Autodesk Inventor part; units mm, degrees
ref_plane "YZ Plane" through (0, 0, 0) normal (1, 0, 0) x (0, 1, 0)
ref_plane "XZ Plane" through (0, 0, 0) normal (0, 1, 0) x (-1, 0, 0)
ref_plane "XY Plane" through (0, 0, 0) normal (0, 0, 1) x (1, 0, 0)
sketch "スケッチ1" plane through (0, 0, 0) normal (0, 0, 1) x (1, 0, 0)
  arc A0 (149.5249, 111.6966) -> (149.4642, 111.5067) centre (150.3865, 111.3165) ccw
  arc A1 (149.9412, 112.3564) -> (149.5249, 111.6966) centre (151.9548, 110.6246) ccw
  arc A2 (151.4141, 113.5151) -> (149.9412, 112.3564) centre (153.6271, 109.1863) ccw
  arc A3 (143.9033, 109.9765) -> (144.0139, 109.8107) centre (144.7377, 110.4132) ccw
  arc A4 (143.647, 110.7134) -> (143.9033, 109.9765) centre (146.2564, 111.2079) ccw
  arc A5 (143.6595, 112.5874) -> (143.647, 110.7134) centre (148.4237, 111.6186) ccw
  arc A6 (141.7431, 104.509) -> (141.9418, 104.492) centre (141.922, 105.4335) ccw
  arc A7 (141.0072, 104.768) -> (141.7431, 104.509) centre (142.2475, 107.1165) ccw
  arc A8 (139.5499, 105.9462) -> (141.0072, 104.768) centre (143.2777, 109.0669) ccw
  arc A9 (144.671, 99.4111) -> (144.8081, 99.5559) centre (144.0597, 100.1274) ccw
  arc A10 (144.0096, 98.9973) -> (144.671, 99.4111) centre (142.9469, 101.4312) ccw
  arc A11 (142.1798, 98.5924) -> (144.0096, 98.9973) centre (142.0642, 103.4527) ccw
  arc A12 (150.4822, 98.5217) -> (150.4545, 98.7192) centre (149.541, 98.4903) ccw
  arc A13 (150.3933, 97.7466) -> (150.4822, 98.5217) centre (147.8278, 98.4333) ccw
  arc A14 (149.569, 96.0636) -> (150.3933, 97.7466) centre (145.697, 99.0035) ccw
  arc A15 (154.8007, 102.5106) -> (154.6291, 102.612) centre (154.2384, 101.7552) ccw
  arc A16 (155.3513, 101.9579) -> (154.8007, 102.5106) centre (153.2149, 100.3801) ccw
  arc A17 (156.1532, 100.264) -> (155.3513, 101.9579) centre (151.4405, 99.0698) ccw
  arc A18 (154.3747, 108.3739) -> (154.1884, 108.303) centre (154.6147, 107.4633) ccw
  arc A19 (155.1501, 108.4598) -> (154.3747, 108.3739) centre (155.0516, 105.8058) ccw
  arc A20 (156.9743, 108.0306) -> (155.1501, 108.4598) centre (154.9697, 103.6015) ccw
  arc A21 (147.5358, 111.5067) -> (147.4751, 111.6966) centre (146.6135, 111.3165) ccw
  arc A22 (147.4751, 111.6966) -> (147.0588, 112.3564) centre (145.0452, 110.6246) ccw
  arc A23 (147.0588, 112.3564) -> (145.5858, 113.5151) centre (143.3729, 109.1863) ccw
  arc A24 (142.8116, 108.303) -> (142.6253, 108.3739) centre (142.3853, 107.4633) ccw
  arc A25 (142.6253, 108.3739) -> (141.8499, 108.4598) centre (141.9484, 105.8058) ccw
  arc A26 (141.8499, 108.4598) -> (140.0256, 108.0306) centre (142.0302, 103.6015) ccw
  arc A27 (142.3709, 102.612) -> (142.1993, 102.5106) centre (142.7615, 101.7552) ccw
  arc A28 (142.1993, 102.5106) -> (141.6486, 101.9579) centre (143.7851, 100.3801) ccw
  arc A29 (141.6486, 101.9579) -> (140.8468, 100.264) centre (145.5595, 99.0698) ccw
  arc A30 (146.5455, 98.7192) -> (146.5178, 98.5217) centre (147.459, 98.4903) ccw
  arc A31 (146.5178, 98.5217) -> (146.6066, 97.7466) centre (149.1722, 98.4333) ccw
  arc A32 (146.6066, 97.7466) -> (147.431, 96.0636) centre (151.303, 99.0035) ccw
  arc A33 (152.1919, 99.5559) -> (152.329, 99.4111) centre (152.9403, 100.1274) ccw
  arc A34 (152.329, 99.4111) -> (152.9903, 98.9973) centre (154.0531, 101.4312) ccw
  arc A35 (152.9903, 98.9973) -> (154.8201, 98.5924) centre (154.9358, 103.4527) ccw
  arc A36 (155.0582, 104.492) -> (155.2568, 104.509) centre (155.078, 105.4335) ccw
  arc A37 (155.2568, 104.509) -> (155.9927, 104.768) centre (154.7524, 107.1165) ccw
  arc A38 (155.9927, 104.768) -> (157.4501, 105.9462) centre (153.7223, 109.0669) ccw
  arc A39 (152.986, 109.8107) -> (153.0967, 109.9765) centre (152.2623, 110.4132) ccw
  arc A40 (153.0967, 109.9765) -> (153.3529, 110.7134) centre (150.7435, 111.2079) ccw
  arc A41 (153.3529, 110.7134) -> (153.3404, 112.5874) centre (148.5763, 111.6186) ccw
  arc A42 (149.3355, 110.6383) -> (147.6645, 110.6383) centre (148.5, 104.9999) ccw
  arc A43 (144.6126, 109.1687) -> (143.5707, 107.8622) centre (148.5, 104.9999) ccw
  arc A44 (142.817, 104.5598) -> (143.1888, 102.9307) centre (148.5, 104.9999) ccw
  arc A45 (145.3008, 100.2824) -> (146.8063, 99.5573) centre (148.5, 104.9999) ccw
  arc A46 (150.1936, 99.5573) -> (151.6992, 100.2824) centre (148.5, 104.9999) ccw
  arc A47 (153.8111, 102.9307) -> (154.183, 104.5598) centre (148.5, 104.9999) ccw
  arc A48 (153.4292, 107.8622) -> (152.3873, 109.1687) centre (148.5, 104.9999) ccw
  arc A49 (145.5858, 113.5151) -> (143.6595, 112.5874) centre (148.5, 104.9999) ccw
  arc A50 (140.0256, 108.0306) -> (139.5499, 105.9462) centre (148.5, 104.9999) ccw
  arc A51 (140.8468, 100.264) -> (142.1798, 98.5924) centre (148.5, 104.9999) ccw
  arc A52 (147.431, 96.0636) -> (149.569, 96.0636) centre (148.5, 104.9999) ccw
  arc A53 (154.8201, 98.5924) -> (156.1532, 100.264) centre (148.5, 104.9999) ccw
  arc A54 (157.4501, 105.9462) -> (156.9743, 108.0306) centre (148.5, 104.9999) ccw
  arc A55 (153.3404, 112.5874) -> (151.4141, 113.5151) centre (148.5, 104.9999) ccw
  line L0 (149.3355, 110.6383) -> (149.4642, 111.5067)
  line L1 (144.6126, 109.1687) -> (144.0139, 109.8107)
  line L2 (142.817, 104.5598) -> (141.9418, 104.492)
  line L3 (145.3008, 100.2824) -> (144.8081, 99.5559)
  line L4 (150.1936, 99.5573) -> (150.4545, 98.7192)
  line L5 (153.8111, 102.9307) -> (154.6291, 102.612)
  line L6 (153.4292, 107.8622) -> (154.1884, 108.303)
  line L7 (147.6645, 110.6383) -> (147.5358, 111.5067)
  line L8 (143.5707, 107.8622) -> (142.8116, 108.303)
  line L9 (143.1888, 102.9307) -> (142.3709, 102.612)
  line L10 (146.8063, 99.5573) -> (146.5455, 98.7192)
  line L11 (151.6992, 100.2824) -> (152.1919, 99.5559)
  line L12 (154.183, 104.5598) -> (155.0582, 104.492)
  line L13 (152.3873, 109.1687) -> (152.986, 109.8107)
  line L14 (137.5, 105) -> (159.5, 105)
  line L15 (148.5, 94) -> (148.5, 116)
  line L16 (177.5, 113.9999) -> (247.5, 113.9999)
  line L17 (177.5, 105.9999) -> (247.5, 105.9999)
  line L18 (177.5, 97.9999) -> (247.5, 97.9999)
  line L19 (177.5, 89.9999) -> (247.5, 89.9999)
  line L20 (177.5, 81.9999) -> (247.5, 81.9999)
  line L21 (177.5, 73.9999) -> (247.5, 73.9999)
  line L22 (177.5, 65.9999) -> (247.5, 65.9999)
  line L23 (177.5, 57.9999) -> (247.5, 57.9999)
  line L24 (177.5, 49.9999) -> (247.5, 49.9999)
  line L25 (177.5, 41.9999) -> (247.5, 41.9999)
  line L26 (177.5, 33.9999) -> (247.5, 33.9999)
  line L27 (177.5, 25.9999) -> (247.5, 25.9999)
  line L28 (177.5, 17.9999) -> (247.5, 17.9999)
  line L29 (177.5, 113.9999) -> (177.5, 17.9999)
  line L30 (247.5, 113.9999) -> (247.5, 17.9999)
  line L31 (212.5, 105.9999) -> (212.5, 17.9999)
  arc A56 (151.9641, 105.75) -> (150.8816, 107.625) centre (150.8816, 106.375) ccw
  arc A57 (151.9641, 105.75) -> (151.9641, 104.25) centre (153.2631, 105) ccw
  arc A58 (150.8816, 102.375) -> (151.9641, 104.25) centre (150.8816, 103.625) ccw
  arc A59 (147.4175, 101.625) -> (149.5825, 101.625) centre (148.5, 102.25) ccw
  arc A60 (150.8816, 102.375) -> (149.5825, 101.625) centre (150.8816, 100.875) ccw
  arc A61 (147.4175, 101.625) -> (146.1184, 102.375) centre (146.1184, 100.875) ccw
  arc A62 (146.1184, 107.625) -> (145.0359, 105.75) centre (146.1184, 106.375) ccw
  arc A63 (146.1184, 107.625) -> (147.4175, 108.375) centre (146.1184, 109.125) ccw
  line L32 (145.0359, 107) -> (148.5, 109) construction
  circle A64 centre (148.5, 105) radius 5 construction
  arc A65 (149.5825, 108.375) -> (147.4175, 108.375) centre (148.5, 107.75) ccw
  arc A66 (145.0359, 104.25) -> (145.0359, 105.75) centre (143.7369, 105) ccw
  arc A67 (149.5825, 108.375) -> (150.8816, 107.625) centre (150.8816, 109.125) ccw
  line L33 (145.0359, 103) -> (145.0359, 107) construction
  arc A68 (145.0359, 104.25) -> (146.1184, 102.375) centre (146.1184, 103.625) ccw
  line L34 (148.5, 109) -> (151.9641, 107) construction
  line L35 (148.5, 101) -> (145.0359, 103) construction
  circle A69 centre (148.5, 105) radius 4 construction
  circle A70 centre (148.5, 105) radius 3.2631 construction
  line L36 (151.9641, 103) -> (148.5, 101) construction
  line L37 (151.9641, 107) -> (151.9641, 103) construction
  circle A71 centre (148.5, 105) radius 2.025
  point P0 (0, 0)
  point P1 (183.5, 108)
  point P2 (186, 100)
  point P3 (186, 92)
  point P4 (183.5, 84)
  point P5 (186, 76)
  point P6 (181, 68)
  point P7 (183.5, 60)
  point P8 (183.5, 52)
  point P9 (183.5, 44)
  point P10 (186, 36)
  point P11 (186, 28)
  point P12 (183.5, 20)
  point P13 (213.5, 100)
  point P14 (229.75, 92)
  point P15 (229.75, 84)
  point P16 (226, 76)
  point P17 (228.5, 68)
  point P18 (222.25, 60)
  point P19 (228.5, 52)
  point P20 (226, 44)
  point P21 (223.5, 36)
  point P22 (231, 28)
  point P23 (231, 20)
  point P24 (149.5, 129.5)
  point P25 (149.5, 123.5)
  point P26 (166.75, 129.5)
  point P27 (168.875, 123.5)
  point P28 (151.9641, 107)
  point P29 (151.9641, 103)
  point P30 (148.5, 101)
  point P31 (145.0359, 103)
  point P32 (151.9641, 105.75)
  point P33 (151.9641, 104.25)
  point P34 (150.8816, 102.375)
  point P35 (149.5825, 101.625)
  point P36 (147.4175, 101.625)
  point P37 (146.1184, 102.375)
  point P38 (145.0359, 104.25)
  point P39 (145.0359, 105.75)
  point P40 (146.1184, 107.625)
  dimension "d5" = 8
  dimension "d4" = 10
  dimension "d6" = 360
  dimension "d7" = 360
  dimension "d8" = 6.5263
  dimension "d9" = 1.5
  dimension "d10" = 1.25
  dimension "d11" = 4.05
extrude "押し出し1" add sketch "スケッチ1" along normal blind 5.9 contours A1 A2 A55 A41 A40 A39 L13 A48 L6 A18 A19 A20 A54 A38 L14 A57 A56 A67 A65 L15 A42 L0 A0 | L15 A65 A63 A62 A66 L14 A8 A50 A26 A25 A24 L8 A43 L1 A3 A4 A5 A49 A23 A22 A21 L7 A42 | L14 A38 A37 A36 L12 A47 L5 A15 A16 A17 A53 A35 A34 A33 L11 A46 L4 A12 A13 A14 A52 L15 A59 A60 A58 A57 | A66 A68 A61 A59 L15 A52 A32 A31 A30 L10 A45 L3 A9 A10 A11 A51 A29 A28 A27 L9 A44 L2 A6 A7 A8 L14
extrude "押し出し2" add sketch "スケッチ1" along normal blind 3.3 contours A65 A67 A56 A57 L14 A71 L15 | L15 A71 L14 A66 A62 A63 A65 | L14 A57 A58 A60 A59 L15 A71 | A71 L15 A59 A61 A68 A66 L14
properties part number "m2z7" material "アルミニウム 2014-T4"
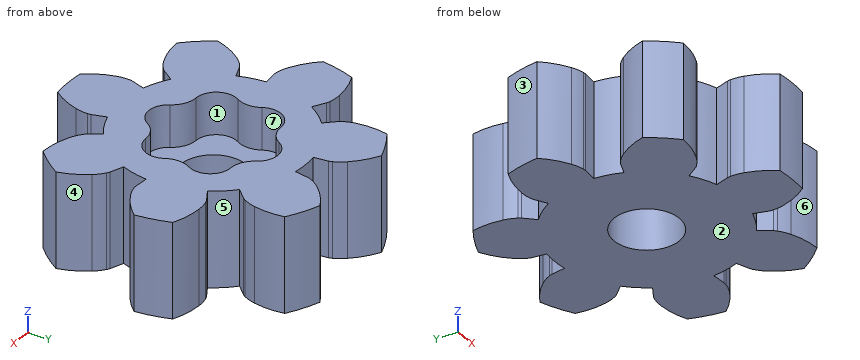
Build history of the part. All positions in model axes, mm. Face numbers are marked on the shaded views. A direction names the side the tool comes from. Round coordinates to 2 decimals unless told otherwise and drop trailing zeros. Write each loop counter-clockwise with the first axis right and the second up, starting at its lowest first coordinate (ties: lowest second). Pieces come first, ordered by that corner, then holes. Notation, with made-up numbers: (18, 27) - (59, 27) arc R23 cw to (59, 38) - close; hole circle Ø3 at (38.25, 72.25). An arc over 180 degrees is marked (long way). Write each question's results on one line, items separated by ' | '. Start each with the question number.
Item 1: Mould opens along X. For the marked faces 1, 2 and 3 say: pulls with the +X half, pulls with the -X half, needs draft (parallel to the pull), parting line crosses it, or undercut.
Item 2: Saw through at B-B (x = 148.5). Write the cut outline in (y, z) (3 decimals), and give its area (3 significant figures).
Item 3: Saw through at C-C (y = 112). Write the cut outline in (x, z).
Item 4: Saw through at A-A (y = 105). Write the cut outline in (x, z) (3 decimals).
Item 5: Wall check: L1, parallel to X at y = 99.75, z = 4.05; L2, parallel to Y at x = 148.5, z = 2.2 (3 decimals); L3, parallel to X at y = 105, z = 2.35 (3 decimals). Give the ranges that are in metal, low to high. Write a range as [from, to].
Item 6: Which spindle directions (+Z, -Z, +X, -X, +Y, -Y) get a long thin tool onto all of the face, cutting with end or side? Do the marked faces 4, 5, 6 and 7. Say none if no direction does.
Item 7: Drop flat-ended pins along their axis: P1, Ø1.5, axis at y = 111.5, z = 3, coming from the +X side; P2, Ø4.5, axis at x = 148.5, y = 105, coming from the +Z side. Give the stop position or say it passes through.
Results are:
1) face 1: undercut | face 2: needs draft | face 3: pulls with the -X half
2) outline: (96, 0) - (102.975, 0) - (102.975, 3.3) - (101, 3.3) - (101, 5.9) - (96, 5.9) - close; (107.025, 0) - (110.7, 0) - (110.7, 5.9) - (109, 5.9) - (109, 3.3) - (107.025, 3.3) - close | area: 52.6 mm²
3) outline: (143.58, 0) - (147.32, 0) - (147.32, 5.9) - (143.58, 5.9) - close; (149.68, 0) - (153.42, 0) - (153.42, 5.9) - (149.68, 5.9) - close
4) outline: (140.614, 0) - (146.475, 0) - (146.475, 3.3) - (145.237, 3.3) - (145.237, 5.9) - (140.614, 5.9) - close; (150.525, 0) - (156.386, 0) - (156.386, 5.9) - (151.763, 5.9) - (151.763, 3.3) - (150.525, 3.3) - close
5) L1: x = [141.19, 144.94], [146.28, 150.72], [152.06, 155.81] | L2: y = [96, 102.975], [107.025, 110.7] | L3: x = [140.614, 146.475], [150.525, 156.386]
6) face 4: +Z, -Z, +X | face 5: +Z, -Z | face 6: +Z, -Z, -Y | face 7: +Z
7) P1: stops at x = 153.44 | P2: stops at z = 3.3
